from build123d import *

# Parameters (mm, degrees)
SKETCH1_R               = 190.5
BOSS_EXTRUDE1_DEPTH     = 25.4
SKETCH2_R               = 184.15
CUT_EXTRUDE1_DEPTH      = 25.4
CUT_EXTRUDE2_REACH      = 272.602
CUT_EXTRUDE2_END_RADIUS = 190.5
SKETCH3_W               = 50.8
SKETCH3_H               = 19.05


with BuildPart() as part:
    # Sketch1 → Boss-Extrude1 (new body)
    with BuildSketch(Plane.XY):
        Circle(SKETCH1_R)
    extrude(amount=BOSS_EXTRUDE1_DEPTH)

    # Sketch2 → Cut-Extrude1 (cut)
    with BuildSketch(Plane.XY.offset(25.4)):
        Circle(SKETCH2_R)
    extrude(amount=-CUT_EXTRUDE1_DEPTH, mode=Mode.SUBTRACT)

    # Cut-Extrude2: up to this cylinder (the profile starts inside it)
    cut_extrude2_end = Plane(origin=(0, 0, 12.7), z_dir=(0, 0, -1)) * Cylinder(CUT_EXTRUDE2_END_RADIUS, 927.204, mode=Mode.PRIVATE)
    # Sketch3 → Cut-Extrude2 (cut, up to the surface)
    with BuildSketch(Plane(origin=(0, 0, 0), x_dir=(1, 0, 0), z_dir=(0, 1, 0)), mode=Mode.PRIVATE) as cut_extrude2_sk1:
        with Locations((3.83525529, -12.7)):
            Rectangle(SKETCH3_W, SKETCH3_H)
    cut_extrude2_tool1 = extrude(cut_extrude2_sk1.sketch, amount=-CUT_EXTRUDE2_REACH, mode=Mode.PRIVATE) & cut_extrude2_end
    add(cut_extrude2_tool1.solids().sort_by_distance((3.835255, 0, 12.7))[0], mode=Mode.SUBTRACT)


solid = part.part
The listing builds one solid part. Answer for the finished solid, in the listing's coordinates (mm). A direction names the side the tool comes from. Coordinates: 2 decimals unless noted, no trailing zeros. Order: outer loops, then holes, each group sorted by start corner. A loop starts at its lowest first (then second) coordinate and runs counter-clockwise, first axis right, second up. Notation, with made-up numbers: (-4.5, 49) -> (46.5, 49) arc R9 ccw to (46.5, 63) -> close; hole circle Ø9 at (77, -19.75). An arc over 180 degrees is marked (long way). Answer in a Markdown table with one row per item. Add a question column.
Item 1: Find section D-D (z = 8.5). Write down the section's boundary in (x, y).
Item 2: Find section A-A (x = 0). Write down the section's boundary in (y, z) (3 decimals), then the cut area to 3 significant figures.
Item 3: Find section B-B (y = 0). Write down the section's boundary in (x, z).
Item 4: Determine the mould class of faces 3 (the face through (-100, 156, 0)), 4 (the face through (-100, 156, 25.4)), 5 (the face through (3, -187, 3.175)) for opening direction Z: +Z half, -Z half, draft (parallel to the pull), parting line (faces both ways), or undercut.
Item 5: Which of the six approach directions +Z, -Z, +X, -X, +Y, -Y give full straight-line access (tool end or side, diameter ignored) to faces 1 (the face through (3, -187, 22.225)), 2 (the face through (-146.1, -112.1, 12.9))?
Item 6: Find section C-C (y = -133.5). Write down the section's boundary in (x, z), then the cut area to 3 significant figures.
Item 7: Each of these flat-tipped pins is pushed along its axis until it touches: P1, Ø12, axis at y = -99, z = 10.5, coming from the -X side; P2, Ø2, axis at y = -69, z = 13.5, coming from the +X side; P3, Ø1.5, axis at x = 148.5, z = 22, coming from the -Y side. Where does it stop, or does it pass through?
Item 8: Find the intervals of material crossed by L1, parallel to Y at x = 0, z = 18.75; L2, parallel to Y at x = -102.5, z = 23; L3, parallel to X at y = -137.5, z = 21.5, in increasing order. Write a range as from..to.
Result set:
| question | item | result |
|---|---|---|
| 1 | outline | (-21.56, -189.28) -> (-21.56, -182.88) arc R184.15 cw (long way) to (29.24, -181.81) -> (29.24, -188.24) arc R190.5 ccw (long way) to start |
| 2 | outline | (-190.5, 0) -> (-184.15, 0) -> (-184.15, 3.175) -> (-190.5, 3.175) -> close; (-190.5, 22.225) -> (-184.15, 22.225) -> (-184.15, 25.4) -> (-190.5, 25.4) -> close; (184.15, 0) -> (190.5, 0) -> (190.5, 25.4) -> (184.15, 25.4) -> close |
| 2 | area | 202 mm² |
| 3 | outline | (-190.5, 0) -> (-184.15, 0) -> (-184.15, 25.4) -> (-190.5, 25.4) -> close; (184.15, 0) -> (190.5, 0) -> (190.5, 25.4) -> (184.15, 25.4) -> close |
| 4 | face 3 | -Z half |
| 4 | face 4 | +Z half |
| 4 | face 5 | undercut |
| 5 | face 1 | -Y |
| 5 | face 2 | +Z, -Z |
| 6 | outline | (-135.9, 0) -> (-126.84, 0) -> (-126.84, 25.4) -> (-135.9, 25.4) -> close; (126.84, 0) -> (135.9, 0) -> (135.9, 25.4) -> (126.84, 25.4) -> close |
| 6 | area | 460 mm² |
| 7 | P1 | stops at x = -166.26 |
| 7 | P2 | stops at x = 177.95 |
| 7 | P3 | stops at y = -120.25 |
| 8 | L1 | y = 184.15..190.5 |
| 8 | L2 | y = -160.57..-152.99, 152.99..160.57 |
| 8 | L3 | x = -131.85..-122.49, 122.49..131.85 |
